Work out the finished part from the listing and answer in its coordinate system (mm). Coordinates: 2 decimals unless noted, no trailing zeros. Write each loop counter-clockwise with the first axis right and the second up, starting at its lowest first coordinate (ties: lowest second). Pieces come first, ordered by that corner, then holes. Notation, with made-up numbers: M 67,-9.5 L 122,-9.5 A23 ccw 122,13.5 Z; hole C 59.5,28.5 d1. An arc over 180 degrees is marked long. Answer as CSV lines item,"result". Start each with the question number.
(1) Find the intervals of material crossed by L1, parallel to X at y = 1.75, z = 48.05; L2, parallel to Z at x = 69.1, y = 1.9; L3, parallel to Z at x = -52, y = 1.3, in increasing order. Write a range as [from, to].
(2) A cutting plane is placed at C-C on x = 54. Give the vertices of the cut face in (y, z).
(3) A cutting plane is placed at A-A on z = -48.05. Give the vertices of the cut face in (x, y).
(4) A cutting plane is placed at B-B on y = 0.85. Give the vertices of the cut face in (x, z), then the cut area to 3 significant figures.
(5) A cutting plane is placed at D-D on z = 27. Give the vertices of the cut face in (x, y), then the cut area to 3 significant figures.
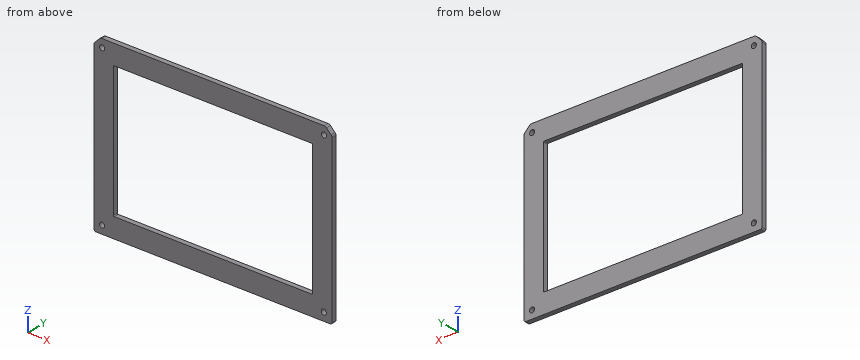
from build123d import *

# Parameters (mm, degrees)
SKETCH1_W           = 148.2
SKETCH1_H           = 106.1
SKETCH1_R           = 1.6
SKETCH1_W_2         = 124.1
SKETCH1_H_2         = 81.8
BOSS_EXTRUDE1_DEPTH = 3
FILLET1_R           = 1
FILLET2_R           = 0.5
CUT_EXTRUDE1_REACH  = 93.182
FILLET3_R           = 2


with BuildPart() as part:
    # Sketch1 → Boss-Extrude1 (new body)
    with BuildSketch(Plane(origin=(0, 0, 0), x_dir=(1, 0, 0), z_dir=(0, 1, 0))):
        Rectangle(SKETCH1_W, SKETCH1_H)
        with Locations(Location((-69.1, 48.05, 0), (0, 0, 270))):
            Circle(SKETCH1_R, mode=Mode.SUBTRACT)
        with Locations(Location((-69.1, -48.05, 0), (0, 0, 90))):
            Circle(SKETCH1_R, mode=Mode.SUBTRACT)
        with Locations(Location((69.1, -48.05, 0), (0, 0, 270))):
            Circle(SKETCH1_R, mode=Mode.SUBTRACT)
        with Locations(Location((69.1, 48.05, 0), (0, 0, 90))):
            Circle(SKETCH1_R, mode=Mode.SUBTRACT)
        Rectangle(SKETCH1_W_2, SKETCH1_H_2, mode=Mode.SUBTRACT)
    extrude(amount=BOSS_EXTRUDE1_DEPTH)

    # Fillet1
    fillet1_edges = [part.edges().sort_by_distance(p)[0] for p in [
        (-74.1, 1.5, -53.05),
        (74.1, 1.5, -53.05),
        (74.1, 1.5, 53.05),
        (-74.1, 1.5, 53.05),
    ]]
    fillet(fillet1_edges, radius=FILLET1_R)

    # Fillet2
    fillet2_edges = [part.edges().sort_by_distance(p)[0] for p in [
        (62.05, 1.5, 40.9),
        (62.05, 1.5, -40.9),
        (-62.05, 1.5, -40.9),
        (-62.05, 1.5, 40.9),
    ]]
    fillet(fillet2_edges, radius=FILLET2_R)

    # Sketch2 → Cut-Extrude1 (cut, up to next)
    with BuildSketch(Plane(origin=(0, 3, 0), x_dir=(-1, 0, 0), z_dir=(0, 1, 0)), mode=Mode.PRIVATE) as cut_extrude1_sk1:
        Polygon((77.1, 46.05), (67.1, 56.05), (77.1, 56.05), align=None)
    cut_extrude1_tool1 = extrude(cut_extrude1_sk1.sketch, amount=-CUT_EXTRUDE1_REACH, mode=Mode.PRIVATE) & part.part
    # Sketch2 → Cut-Extrude1 (cut, up to next)
    with BuildSketch(Plane(origin=(0, 3, 0), x_dir=(-1, 0, 0), z_dir=(0, 1, 0)), mode=Mode.PRIVATE) as cut_extrude1_sk2:
        Polygon((-77.1, 56.05), (-77.1, 46.05), (-67.1, 56.05), align=None)
    cut_extrude1_tool2 = extrude(cut_extrude1_sk2.sketch, amount=-CUT_EXTRUDE1_REACH, mode=Mode.PRIVATE) & part.part
    add(cut_extrude1_tool1.solids().sort_by_distance((-73.766667, 3, 52.716667))[0], mode=Mode.SUBTRACT)
    add(cut_extrude1_tool2.solids().sort_by_distance((73.766667, 3, 52.716667))[0], mode=Mode.SUBTRACT)

    # Fillet3
    fillet3_edges = [part.edges().sort_by_distance(p)[0] for p in [
        (70.1, 1.5, 53.05),
        (74.1, 1.5, 49.05),
        (-74.1, 1.5, 49.05),
        (-70.1, 1.5, 53.05),
    ]]
    fillet(fillet3_edges, radius=FILLET3_R)


solid = part.part
Here are the results:
1,L1,"x = [-74.1, -70.7], [-67.5, 67.5], [70.7, 74.1]"
1,L2,"z = [-53.05, -49.65], [-46.45, 46.45], [49.65, 53.05]"
1,L3,"z = [-53.05, -40.9], [40.9, 53.05]"
2,outline,"M 0,-53.05 L 3,-53.05 L 3,-40.9 L 0,-40.9 Z; M 0,40.9 L 3,40.9 L 3,53.05 L 0,53.05 Z"
3,outline,"M -74.1,0 L -70.7,0 L -70.7,3 L -74.1,3 Z; M -67.5,0 L 67.5,0 L 67.5,3 L -67.5,3 Z; M 70.7,0 L 74.1,0 L 74.1,3 L 70.7,3 Z"
4,outline,"M -74.1,-52.05 A1 ccw -73.1,-53.05 L 73.1,-53.05 A1 ccw 74.1,-52.05 L 74.1,48.22 A2 ccw 73.51,49.64 L 70.69,52.46 A2 ccw 69.27,53.05 L -69.27,53.05 A2 ccw -70.69,52.46 L -73.51,49.64 A2 ccw -74.1,48.22 Z; hole C -69.1,-48.05 d3.2; hole C -69.1,48.05 d3.2; hole M -62.05,-40.4 A0.5 ccw -61.55,-40.9 L 61.55,-40.9 A0.5 ccw 62.05,-40.4 L 62.05,40.4 A0.5 ccw 61.55,40.9 L -61.55,40.9 A0.5 ccw -62.05,40.4 Z; hole C 69.1,-48.05 d3.2; hole C 69.1,48.05 d3.2"
4,area,"5,520 mm^2"
5,outline,"M -74.1,0 L -62.05,0 L -62.05,3 L -74.1,3 Z; M 62.05,0 L 74.1,0 L 74.1,3 L 62.05,3 Z"
5,area,"72.3 mm^2"
